Check sheet for the modelled part. Datum: model origin and axes. Units: mm. Coordinates: 2 decimals unless noted, no trailing zeros. Loops run counter-clockwise (first coordinate to the right, second up) from the corner with the lowest first, then second, coordinate; pieces in that order, holes last.
Autodesk Inventor part; units mm, degrees
ref_plane "YZ Plane" through (0, 0, 0) normal (1, 0, 0) x (0, 1, 0)
ref_plane "XZ Plane" through (0, 0, 0) normal (0, 1, 0) x (-1, 0, 0)
ref_plane "XY Plane" through (0, 0, 0) normal (0, 0, 1) x (1, 0, 0)
sketch "Sketch1" plane through (0, 0, 0) normal (0, 1, 0) x (-1, 0, 0)
  arc A0 (210.1622, -7.2025) -> (309.6615, 148.1866) centre (370, 0) ccw construction
  line L0 (370, 0) -> (223.7542, 20.1499)
  circle A1 centre (211.4974, 21.8387) radius 160 construction
  circle A2 centre (369.9872, 0.0018) radius 3 construction
  line L1 (365.7713, 2.7478) -> (370.7713, 2.7478)
  line L2 (370.7713, 2.7478) -> (370.7713, -2.2522)
  line L3 (370.7713, -2.2522) -> (365.7713, -2.2522)
  line L4 (365.7713, -2.2522) -> (365.7713, 2.7478)
  arc A3 (216.7601, 17.6252) -> (215.9023, -5.0762) centre (229.7182, 5.7687) ccw
  circle A4 centre (229.7182, 5.7687) radius 11.5
  circle A5 centre (229.7182, 5.7687) radius 4
  spline S0 degree 4 poles (229.7182, -7.8653) (241.4545, -7.4272) (257.5169, -6.7771) (277.3318, -5.8971) (299.9482, -4.5961) (314.7433, -3.6129) (328.1612, -2.6484) (339.8268, -1.769) (350.012, -1.0496) (357.5866, -0.5225) (364.806, -0.1794) (367.4848, -0.031) (370.1657, -0.0078) (369.9872, 0.0018) knots 0 0 0 0 0 0.270374 0.37387 0.473524 0.56865 0.658428 0.741816 0.817434 0.88334 0.936143 1 1 1 1 1
  arc A6 (223.7542, 20.1499) -> (216.7601, 17.6252) centre (222.6622, 12.2248) ccw
  arc A7 (215.9023, -5.0762) -> (222.4776, -8.1316) centre (222.1952, -0.1366) ccw
  line L5 (222.4776, -8.1316) -> (229.7182, -7.8653)
  point P0 (370, 0)
  point P1 (210.0997, -8.5616)
  point P2 (267.1071, -6.3194)
  point P3 (284.4371, -5.4606)
  point P4 (300.619, -4.5258)
  point P5 (315.5184, -3.5432)
  point P6 (328.988, -2.5786)
  point P7 (340.8625, -1.7041)
  point P8 (350.9622, -0.9861)
  point P9 (359.0984, -0.4682)
  point P10 (365.0855, -0.1602)
  point P11 (368.7597, -0.0285)
  point P12 (368.4073, 0.2194)
  point P13 (365.7713, 0.5826)
  point P14 (220.3414, 20.6201)
  point P15 (365.7713, -0.1283)
  dimension "d5" = 160
  dimension "d25" = 6
  dimension "d26" = 5
  dimension "d27" = 5
  dimension "d41" = 23
  dimension "d60" = 8
  dimension "d65" = 8
extrude "Extrusion4" add sketch "Sketch1" along normal blind 2.5 contours S0 L5 A7 A3 A6 L0 L4 | A4
properties part number "airfoil blueprint"
1) Depth check by flat-ended pin: pin 1 (1.5 mm diameter, centred on y = 2, z = 8.5, fed in from +X). Enter the tip coordinate at first touch or a pass-through.
Answer sheet:
pin 1: stops at x = -212.27
2) Section check A-A on z = 3.25. Enter the section's corners in (x, y), plus the area to 3 significant figures.
Answer sheet:
outline: (-346.41, 0) - (-232.83, 0) - (-232.83, 2.5) - (-346.41, 2.5) - close; (-226.61, 0) - (-212.34, 0) - (-212.34, 2.5) - (-226.61, 2.5) - close
area: 320 mm2
3) Mould release check, pull along Z, two halves, no side actions. Record for faces 1 (the flat face through (-271, 0, 3)), 2 (the cylindrical face through (-233.533, 1.232, 4.567)), 3 (the flat face through (-226.05, 1.23, -8)): +Z half, -Z half, draft (parallel to the pull), parting line (faces both ways), or undercut.
Answer sheet:
face 1: draft
face 2: undercut
face 3: -Z half
4) Scan lines: line 1 (Z direction, x = -230.5, y = 1.95); line 2 (Z direction, x = -243.5, y = 1.9); line 3 (Z direction, x = -302.5, y = 1.7). Record each from-to range of solid material in increasing order.
Answer sheet:
line 1: z = -7.84 to 1.85, 9.69 to 19.22
line 2: z = -7.33 to 17.43
line 3: z = -4.41 to 9.3
